```python
from build123d import *

# Parameters (mm, degrees)
SKETCH1_R           = 14.2875
BOSS_EXTRUDE2_DEPTH = 12.7
SKETCH3_R           = 3.175
CUT_EXTRUDE2_DEPTH  = 12.7


with BuildPart() as part:
    # Sketch1 → Boss-Extrude2 (new body)
    with BuildSketch(Plane.XY):
        with BuildLine():
            Line((50.8, 50.8), (0, 50.8))
            Line((0, 50.8), (-6.517989108, 32.237254305))
            ThreePointArc((-6.517989108, 32.237254305), (-5.465821228, 16.093196457), (6.906112814, 5.668566529))
            Line((6.906112814, 5.668566529), (23.580878621, 0.557579402))
            ThreePointArc((23.580878621, 0.557579402), (25.420999377, 0.140168361), (27.302655351, 0))
            Line((27.302655351, 0), (50.8, 0))
            Line((50.8, 0), (50.8, 50.8))
        make_face()
        with Locations((12.954, 25.4)):
            Circle(SKETCH1_R, mode=Mode.SUBTRACT)
    extrude(amount=BOSS_EXTRUDE2_DEPTH)

    # Sketch3 → Cut-Extrude2 (cut)
    with BuildSketch(Plane(origin=(0, 50.8, 0), x_dir=(1, 0, 0), z_dir=(0, 1, 0))):
        with Locations((45.085, -6.35)):
            Circle(SKETCH3_R)
        with Locations((5.715, -6.35)):
            Circle(SKETCH3_R)
    extrude(amount=-CUT_EXTRUDE2_DEPTH, mode=Mode.SUBTRACT)


solid = part.part
```
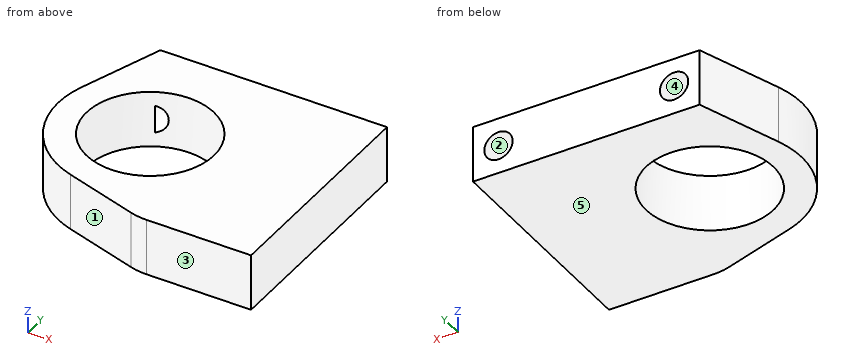
The model under review builds one solid part; all positions refer to its coordinate system, in mm. Face numbers are marked on the shaded views. A direction names the side the tool comes from. Round coordinates to 2 decimals unless told otherwise and drop trailing zeros. Loops run counter-clockwise (first coordinate to the right, second up) from the corner with the lowest first, then second, coordinate; pieces in that order, holes last. Notation, with made-up numbers: (-21.5, 4.25) - (11.5, 4.25) arc R12 cw to (11.5, 16.25) - close; hole circle Ø5 at (49, 29.5). An arc over 180 degrees is marked (long way). Write each question's results on one line, items separated by ' | '. Start each with the question number.
Q1. Insertion check: P1, Ø6, axis at x = 13, z = 10.5, coming from the -Y side; P2, Ø1.9, axis at x = 45.5, z = 5.5, coming from the +Y side; P3, Ø5.5, axis at x = 5.715, z = 6.35, coming from the -Y side. Each pin has a flat end and moves straight along its axis. Give the tip position at first contact, or say it passes through.
Q2. Wall thickness on line 1 along X through (y, z) = (40.5, 6.35); line 2 along Z through (x, y) = (45, 42.5); line 3 along X through (y, z) = (24.5, 5.25): over which ranges is each line inside the solid? List them lowest first. Write a range as [from, to].
Q3. Take a section at D-D on z = 6.35. Give the boundary of the cut face in (x, y) (1 decimal), plus the area to 3 significant figures.
Q4. Take a section at C-C on x = 15. Give the boundary of the cut face in (y, z).
Q5. Draft analysis for pull direction X (two halves, no side actions). For the marked faces 1, 2 and 3, state which applies: pulls with the +X half, pulls with the -X half, needs draft (parallel to the pull), parting line crosses it, or undercut.
Q6. Take a section at A-A on y = 37. Give the boundary of the cut face in (x, z).
Q7. Tool access review of the marked faces 4 and 5: name each direction out of +Z, -Z, +X, -X, +Y, -Y from which nothing blocks a thin tool from reaching the whole face with its end or side.
Q8. Take a section at B-B on z = 10.25. Give the boundary of the cut face in (x, y) (1 decimal).
Data:
1) P1: stops at y = 2.88 | P2: stops at y = 38.1 | P3: stops at y = 5.19
2) line 1: x = [-3.62, 2.54], [8.89, 41.91], [48.26, 50.8] | line 2: z = [0, 3.18], [9.52, 12.7] | line 3: x = [-7.66, -1.31], [27.21, 50.8]
3) outline: (-6.5, 32.2) arc R20.6 ccw to (6.9, 5.7) - (23.6, 0.6) arc R12.7 ccw to (27.3, 0) - (50.8, 0) - (50.8, 50.8) - (48.3, 50.8) - (48.3, 38.1) - (41.9, 38.1) - (41.9, 50.8) - (8.9, 50.8) - (8.9, 39.1) arc R14.3 cw (long way) to (6.4, 38.1) - (2.5, 38.1) - (2.5, 50.8) - (0, 50.8) - close | area: 1,870 mm²
4) outline: (3.19, 0) - (11.26, 0) - (11.26, 12.7) - (3.19, 12.7) - close; (39.54, 0) - (50.8, 0) - (50.8, 12.7) - (39.54, 12.7) - close
5) face 1: pulls with the -X half | face 2: undercut | face 3: needs draft
6) outline: (-4.85, 0) - (4.61, 0) - (4.61, 12.7) - (-4.85, 12.7) - close; (21.3, 0) - (50.8, 0) - (50.8, 12.7) - (21.3, 12.7) - close
7) face 4: +Y | face 5: -Z, +X, -X, +Y, -Y
8) outline: (-6.5, 32.2) arc R20.6 ccw to (6.9, 5.7) - (23.6, 0.6) arc R12.7 ccw to (27.3, 0) - (50.8, 0) - (50.8, 50.8) - (0, 50.8) - close; hole circle Ø28.6 at (13, 25.4)
